Input: part model. Units: mm. Frame: model coordinates. A direction names the side the tool comes from. Give positions to 0.01 mm unless a question says otherwise; leave off trailing zeros. Write each loop counter-clockwise with the first axis right and the second up, starting at its lowest first coordinate (ties: lowest second). Pieces come first, ordered by that corner, then holes.
```python
from build123d import *

# Parameters (mm, degrees)
CYLINDER018_R                              = 1.4
CYLINDER018_DEPTH                          = 27
CYLINDER020_R                              = 2
CYLINDER020_DEPTH                          = 8
CYLINDER021_R                              = 2
CYLINDER021_DEPTH                          = 8
CYLINDER019_R                              = 1.4
CYLINDER019_DEPTH                          = 27
CYLINDER017_R                              = 10
CYLINDER017_DEPTH                          = 81.5
CHAMFER004013007011015006009007001084_SIZE = 0.4


with BuildPart() as cylinder018:
    # Cylinder018 → Cylinder018 (new body)
    with BuildSketch(Plane.XY):
        Circle(CYLINDER018_R)
    extrude(amount=CYLINDER018_DEPTH)


with BuildPart() as cylinder020:
    # Cylinder020 → Cylinder020 (new body)
    with BuildSketch(Plane.XY):
        Circle(CYLINDER020_R)
    extrude(amount=CYLINDER020_DEPTH)


with BuildPart() as cylinder021:
    # Cylinder021 → Cylinder021 (new body)
    with BuildSketch(Plane.XY.offset(73.5)):
        Circle(CYLINDER021_R)
    extrude(amount=CYLINDER021_DEPTH)


with BuildPart() as fusion006002011004053036004001_body:
    # Cylinder019 → Cylinder019 (new body)
    with BuildSketch(Plane.XY.offset(54.5)):
        Circle(CYLINDER019_R)
    extrude(amount=CYLINDER019_DEPTH)

    # Fusion006002011004053036004001028003005014018035002007006012: union Cylinder018, Cylinder020, Cylinder021
    add(cylinder018.part)
    add(cylinder020.part)
    add(cylinder021.part)


with BuildPart() as roller:
    # Cylinder017 → Cylinder017 (new body)
    with BuildSketch(Plane.XY):
        Circle(CYLINDER017_R)
    extrude(amount=CYLINDER017_DEPTH)

    # Cut008004003004014002002005003004003002003021022001002001107: cut Fusion006002011004053036004001 body
    add(fusion006002011004053036004001_body.part, mode=Mode.SUBTRACT)

    # Chamfer004013007011015006009007001084
    chamfer004013007011015006009007001084_edges = [roller.edges().sort_by_distance(p)[0] for p in [
        (-10, 0, 81.5),
        (-10, 0, 0),
        (-2, 0, 81.5),
        (-2, 0, 0),
    ]]
    chamfer(chamfer004013007011015006009007001084_edges, length=CHAMFER004013007011015006009007001084_SIZE)


solid = roller.part
```
Q1. Pin query (flat end, axial travel): pin 1 (3 mm diameter, centred on x = 0, y = 0, fed in from +Z); pin 2 (4.5 mm diameter, centred on x = 0, y = 0, fed in from -Z); pin 3 (2 mm diameter, centred on y = -3, z = 20.5, fed in from -X). Return the tip coordinate at first contact, or that it passes through.
Q2. Section C-C, the plane z = 37. Return the cut outline in (x, y), then the cut area to 3 significant figures.
Q3. Access query for faces 1 (the flat face through (2, -2, 0)), 2 (the flat face through (0, 0, 27)), 3 (the cylindrical face through (0, -2, 77)). Directions: +Z, -Z, +X, -X, +Y, -Y. A direction counts if a zero-diameter tool reaches every point of the face in a straight line with its end or side. Return the directions, or none.
Q4. Section A-A, the plane y = 0. Return the cut outline in (x, z).
Q5. Material intervals for line 1 along Y through (x, z) = (0, 4); line 2 along Y through (x, z) = (0, 12); line 3 along X through (y, z) = (2.75, 34.5), sorted ascending.
Q6. Mould query, pull axis X, two halves, no side actions, for faces 4 (the cylindrical face through (-1.4, 0.06, 63.87)), 5 (the flat face through (2, -2, 81.5)), 6 (the cylindrical face through (-2.17, -9.76, 40.19)). Classes: +X half, -X half, draft (parallel to the pull), parting line (faces both ways), or undercut.
Solutions:
1. pin 1: stops at z = 73.5
1. pin 2: stops at z = 0.15
1. pin 3: stops at x = -9.8
2. outline: circle Ø20 at (0, 0)
2. area: 314 mm2
3. face 1: -Z, +X, -X, +Y, -Y
3. face 2: -Z
3. face 3: +Z
4. outline: (-10, 0.4) - (-9.6, 0) - (-2.4, 0) - (-2, 0.4) - (-2, 8) - (-1.4, 8) - (-1.4, 27) - (1.4, 27) - (1.4, 8) - (2, 8) - (2, 0.4) - (2.4, 0) - (9.6, 0) - (10, 0.4) - (10, 81.1) - (9.6, 81.5) - (2.4, 81.5) - (2, 81.1) - (2, 73.5) - (1.4, 73.5) - (1.4, 54.5) - (-1.4, 54.5) - (-1.4, 73.5) - (-2, 73.5) - (-2, 81.1) - (-2.4, 81.5) - (-9.6, 81.5) - (-10, 81.1) - close
5. line 1: y = -10 to -2, 2 to 10
5. line 2: y = -10 to -1.4, 1.4 to 10
5. line 3: x = -9.61 to 9.61
6. face 4: undercut
6. face 5: draft
6. face 6: parting line
